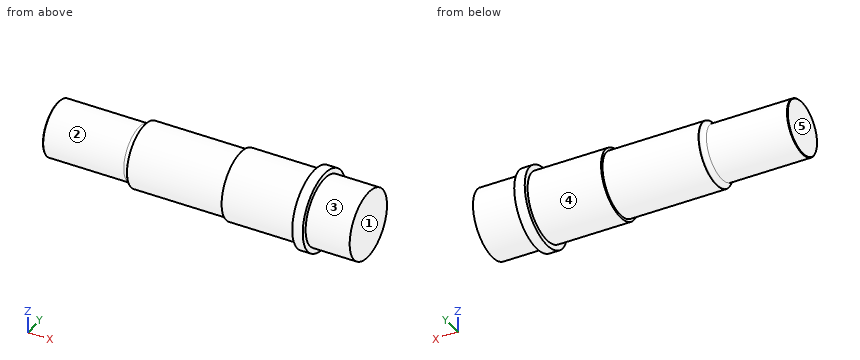
Autodesk Inventor part; units mm, degrees
ref_plane "Начальная плоскость" through (0, 0, 0) normal (1, 0, 0) x (0, 1, 0)
ref_plane "XZ Plane" through (0, 0, 0) normal (0, 1, 0) x (-1, 0, 0)
ref_plane "XY Plane" through (0, 0, 0) normal (0, 0, 1) x (1, 0, 0)
sketch "Основной эскиз" plane through (0, 0, 0) normal (0, 0, 1) x (1, 0, 0)
  line L0 (0, 0) -> (296, 0)
  line L1 (0, 0) -> (0, 26)
  line L2 (0, 26) -> (82, 26)
  line L3 (82, 26) -> (82, 30)
  line L4 (82, 30) -> (174, 30)
  line L5 (174, 30) -> (174, 32.5)
  line L6 (174, 32.5) -> (244, 32.5)
  line L7 (244, 32.5) -> (244, 37.5)
  line L8 (254, 37.5) -> (254, 32.5)
  line L9 (244, 37.5) -> (254, 37.5)
  line L10 (296, 32.5) -> (296, 0)
  line L11 (254, 32.5) -> (296, 32.5)
  dimension "d3" = 52
  dimension "d4" = 60
  dimension "d5" = 65
  dimension "d6" = 75
  dimension "d7" = 65
revolve "Вращение1" add sketch "Основной эскиз" angle 360 about axis through (0, 0, 0) along (1, 0, 0)
chamfer "Фаска3" distance 0.5 angle 45 1 edges at (82, -30, 0) measured on face at (143.3333, 29.9027, -2.414)
chamfer "Фаска1" distance 0.5 angle 45 1 edges at (0, -26, 0) measured on face at (54.6667, 25.9157, -2.0921)
fillet "Сопряжение1" radius 5 1 edges at (82, -26, 0)
equation "\"Length\" = 296"
properties part number "ТихВал" material "Steel"
Here's how the part is built. I have some questions about the finished solid (model axes, mm). Face numbers are marked on the shaded views. A direction names the side the tool comes from. Give positions to 0.01 mm unless a question says otherwise; leave off trailing zeros. Loops run counter-clockwise (first coordinate to the right, second up) from the corner with the lowest first, then second, coordinate; pieces in that order, holes last. Notation, with made-up numbers: M 81.25,80 L 123.25,80 A32 cw 123.25,116 Z; hole C 1.25,22.25 d5. An arc over 180 degrees is marked long. Return JSON: item names as keys, results as strings.
Item 1: I'm going to push flat-ended pins straight in: pin 1 Ø1 at (y, z) = (-27.5, -25.5) entering from -X; pin 2 Ø2 at (x, y) = (262, -6) entering from +Z; pin 3 Ø2 at (x, y) = (59, 28) entering from -Z; pin 4 Ø12 at (x, z) = (214, 18.5) entering from +Y. Where does each tip first touch, or does it pass through?
A:
{"pin 1": "stops at x = 244", "pin 2": "stops at z = 32.11", "pin 3": "passes through", "pin 4": "stops at y = 30"}
Item 2: On a 3-axis mill with a long thin cutter (end or side, diameter ignored), from which of +Z, -Z, +X, -X, +Y, -Y can I reach the whole of each face in a straight line? I mean the marked faces 1, 2 and 3. Say none if no direction works.
A:
{"face 1": "+Z, -Z, +X, +Y, -Y", "face 2": "-X", "face 3": "+X"}
Item 3: Imagine slicing it at C-C on x = 19. List the corners of the cut face in (y, z) for me.
A:
{"outline": "C 0,0 d52"}
Item 4: Please list where these lines run through material, in increasing order: line 1 (X direction, y = 29, z = -10.5); line 2 (X direction, y = 16, z = -33); line 3 (Z direction, x = 41, y = -1.5).
A:
{"line 1": "x = 174 to 296", "line 2": "x = 244 to 254", "line 3": "z = -25.96 to 25.96"}
Item 5: Thinking about a two-plate mould opening in Y: for the marked faces 4 and 5, which applies, released by +Y, released by -Y, zero draft, split by the parting line, or undercut?
A:
{"face 4": "split by the parting line", "face 5": "zero draft"}
Item 6: Imagine slicing it at D-D on x = 272.5. List the corners of the cut face in (y, z) for me.
A:
{"outline": "C 0,0 d65"}
Item 7: Imagine slicing it at A-A on y = 0. List the corners of the cut face in (x, z) for me.
A:
{"outline": "M 0,-25.5 L 0.5,-26 L 77.23,-26 A5 cw 82,-29.5 L 82.5,-30 L 174,-30 L 174,-32.5 L 244,-32.5 L 244,-37.5 L 254,-37.5 L 254,-32.5 L 296,-32.5 L 296,32.5 L 254,32.5 L 254,37.5 L 244,37.5 L 244,32.5 L 174,32.5 L 174,30 L 82.5,30 L 82,29.5 A5 cw 77.23,26 L 0.5,26 L 0,25.5 Z"}
